from build123d import *

# Parameters (mm, degrees)
SKETCH1_W           = 120.65
SKETCH1_H           = 63.5
BOSS_EXTRUDE1_DEPTH = 6.35
CUT_EXTRUDE1_REACH  = 138.488
SKETCH2_W           = 20.32
SKETCH2_H           = 6.35
SKETCH2_W_2         = 41.91


with BuildPart() as part:
    # Sketch1 → Boss-Extrude1 (new body)
    with BuildSketch(Plane.XY):
        with Locations((60.325, 31.75)):
            Rectangle(SKETCH1_W, SKETCH1_H)
    extrude(amount=BOSS_EXTRUDE1_DEPTH)

    # Sketch2 → Cut-Extrude1 (cut, up to next)
    with BuildSketch(Plane.XY.offset(6.35), mode=Mode.PRIVATE) as cut_extrude1_sk1:
        with Locations((16.51, 60.325)):
            Rectangle(SKETCH2_W, SKETCH2_H)
    cut_extrude1_tool1 = extrude(cut_extrude1_sk1.sketch, amount=-CUT_EXTRUDE1_REACH, mode=Mode.PRIVATE) & part.part
    # Sketch2 → Cut-Extrude1 (cut, up to next)
    with BuildSketch(Plane.XY.offset(6.35), mode=Mode.PRIVATE) as cut_extrude1_sk2:
        with Locations((60.325, 60.325)):
            Rectangle(SKETCH2_W_2, SKETCH2_H)
    cut_extrude1_tool2 = extrude(cut_extrude1_sk2.sketch, amount=-CUT_EXTRUDE1_REACH, mode=Mode.PRIVATE) & part.part
    # Sketch2 → Cut-Extrude1 (cut, up to next)
    with BuildSketch(Plane.XY.offset(6.35), mode=Mode.PRIVATE) as cut_extrude1_sk3:
        with Locations((104.14, 60.325)):
            Rectangle(SKETCH2_W, SKETCH2_H)
    cut_extrude1_tool3 = extrude(cut_extrude1_sk3.sketch, amount=-CUT_EXTRUDE1_REACH, mode=Mode.PRIVATE) & part.part
    # Sketch2 → Cut-Extrude1 (cut, up to next)
    with BuildSketch(Plane.XY.offset(6.35), mode=Mode.PRIVATE) as cut_extrude1_sk4:
        with Locations((104.14, 3.175)):
            Rectangle(SKETCH2_W, SKETCH2_H)
    cut_extrude1_tool4 = extrude(cut_extrude1_sk4.sketch, amount=-CUT_EXTRUDE1_REACH, mode=Mode.PRIVATE) & part.part
    # Sketch2 → Cut-Extrude1 (cut, up to next)
    with BuildSketch(Plane.XY.offset(6.35), mode=Mode.PRIVATE) as cut_extrude1_sk5:
        with Locations((60.325, 3.175)):
            Rectangle(SKETCH2_W_2, SKETCH2_H)
    cut_extrude1_tool5 = extrude(cut_extrude1_sk5.sketch, amount=-CUT_EXTRUDE1_REACH, mode=Mode.PRIVATE) & part.part
    # Sketch2 → Cut-Extrude1 (cut, up to next)
    with BuildSketch(Plane.XY.offset(6.35), mode=Mode.PRIVATE) as cut_extrude1_sk6:
        with Locations((16.51, 3.175)):
            Rectangle(SKETCH2_W, SKETCH2_H)
    cut_extrude1_tool6 = extrude(cut_extrude1_sk6.sketch, amount=-CUT_EXTRUDE1_REACH, mode=Mode.PRIVATE) & part.part
    add(cut_extrude1_tool1.solids().sort_by_distance((16.51, 60.325, 6.35))[0], mode=Mode.SUBTRACT)
    add(cut_extrude1_tool2.solids().sort_by_distance((60.325, 60.325, 6.35))[0], mode=Mode.SUBTRACT)
    add(cut_extrude1_tool3.solids().sort_by_distance((104.14, 60.325, 6.35))[0], mode=Mode.SUBTRACT)
    add(cut_extrude1_tool4.solids().sort_by_distance((104.14, 3.175, 6.35))[0], mode=Mode.SUBTRACT)
    add(cut_extrude1_tool5.solids().sort_by_distance((60.325, 3.175, 6.35))[0], mode=Mode.SUBTRACT)
    add(cut_extrude1_tool6.solids().sort_by_distance((16.51, 3.175, 6.35))[0], mode=Mode.SUBTRACT)


solid = part.part
Here's how the part is built. I have some questions about the finished solid (model axes, mm). A direction names the side the tool comes from. Coordinates: 2 decimals unless noted, no trailing zeros. Order: outer loops, then holes, each group sorted by start corner. A loop starts at its lowest first (then second) coordinate and runs counter-clockwise, first axis right, second up. Notation, with made-up numbers: (-17, 82.25) -> (-5, 82.25) arc R20 cw to (-5, 110.25) -> close; hole circle Ø4 at (52.25, 34.5). An arc over 180 degrees is marked (long way). Answer in a Markdown table with one row per item.
(1) I want a section at B-B on x = 75. List the corners of the cut face in (y, z) for me, then the cut area to 3 significant figures.
Answer key:
| item | result |
|---|---|
| outline | (6.35, 0) -> (57.15, 0) -> (57.15, 6.35) -> (6.35, 6.35) -> close |
| area | 323 mm^2 |
(2) Please list where this line runs through material, in increasing order: probe 1 along Y at (x, z) = (53, 5.5).
Answer key:
| item | result |
|---|---|
| probe 1 | 6.35 to 57.15 |
(3) Will these pins go through, and if not, where does the flat tip stop? pin 1 Ø3 at (x, z) = (99, 3) entering from -Y; pin 2 Ø3 at (x, z) = (106.5, 3) entering from +Y; pin 3 Ø2 at (y, z) = (44.5, 5) entering from -X.
Answer key:
| item | result |
|---|---|
| pin 1 | y = 6.35 |
| pin 2 | y = 57.15 |
| pin 3 | x = 0 |
(4) I want a section at A-A on z = 4. List the corners of the cut face in (x, y) for me, then the cut area to 3 significant figures.
Answer key:
| item | result |
|---|---|
| outline | (0, 0) -> (6.35, 0) -> (6.35, 6.35) -> (26.67, 6.35) -> (26.67, 0) -> (39.37, 0) -> (39.37, 6.35) -> (81.28, 6.35) -> (81.28, 0) -> (93.98, 0) -> (93.98, 6.35) -> (114.3, 6.35) -> (114.3, 0) -> (120.65, 0) -> (120.65, 63.5) -> (114.3, 63.5) -> (114.3, 57.15) -> (93.98, 57.15) -> (93.98, 63.5) -> (81.28, 63.5) -> (81.28, 57.15) -> (39.37, 57.15) -> (39.37, 63.5) -> (26.67, 63.5) -> (26.67, 57.15) -> (6.35, 57.15) -> (6.35, 63.5) -> (0, 63.5) -> close |
| area | 6,610 mm^2 |
(5) Thinking about a two-plate mould opening in X: for faces 1 (the face through (39.37, 3, 3)), 2 (the face through (117, 63.5, 3)), which applies, +X half, -X half, draft (parallel to the pull), parting line (faces both ways), or undercut?
Answer key:
| item | result |
|---|---|
| face 1 | undercut |
| face 2 | draft |
(6) On a 3-axis mill with a long thin cutter (end or side, diameter ignored), from which of +Z, -Z, +X, -X, +Y, -Y can I reach the whole of each face in a straight line? I mean faces 3 (the face through (59, 32, 0)), 4 (the face through (114.3, 60, 3)), 5 (the face through (104, 6.35, 3)). Say none if no direction works.
Answer key:
| item | result |
|---|---|
| face 3 | -Z, +X, -X, +Y, -Y |
| face 4 | +Z, -Z, +Y |
| face 5 | +Z, -Z, -Y |
